Build history of the part. All positions in model axes, mm. A direction names the side the tool comes from. Give positions to 0.01 mm unless a question says otherwise; leave off trailing zeros. Loops run counter-clockwise (first coordinate to the right, second up) from the corner with the lowest first, then second, coordinate; pieces in that order, holes last. Notation, with made-up numbers: (21, 40) -> (79, 40) arc R23 ccw to (79, 69) -> close; hole circle Ø3 at (-38, -36). An arc over 180 degrees is marked (long way). Answer as a JSON object with one key per item and string values. Group by question number.
from build123d import *

# Parameters (mm, degrees)
F0_W     = 7.62
F0_H     = 35.56
F1_DEPTH = 10.795
F0_W_2   = 13.335
F2_DEPTH = 6.35
F3_DEPTH = 10.795
F4_DEPTH = 30.48
F5_R     = 3.81
F6_SIZE  = 16.51
F7_R     = 1.524
F8_DEPTH = 76.836
F9_R     = 3.81


# Not quite as in the source:
# - a feature names something its author has since deleted; it is built from what else it names


with BuildPart() as f1:
    # F0 (on Top) → F1 (new body, symmetric)
    with BuildSketch(Plane.XY):
        Polygon((31.75, 44.45), (-31.75, 44.45), (-31.75, 17.78), (-31.75, -17.78), (-31.75, -44.45), (-29.21, -44.45), (31.75, -44.45), (31.75, -31.7187323975), (31.75, -17.78), (31.75, 17.78), align=None)
        with Locations((-25.4, 0)):
            Rectangle(F0_W, F0_H, mode=Mode.SUBTRACT)
        with Locations((25.4, 0)):
            Rectangle(F0_W, F0_H, mode=Mode.SUBTRACT)
    extrude(amount=F1_DEPTH, both=True)



with BuildPart() as f1b:
    # F0 (on Top) → F1, piece 2 (new body, symmetric)
    with BuildSketch(Plane.XY):
        Polygon((-45.085, -17.78), (-45.085, 17.78), (-45.085, 44.45), (-47.625, 44.45), (-47.625, -31.75), (-47.625, -44.45), (-45.085, -44.45), align=None)
    extrude(amount=F1_DEPTH, both=True)


with BuildPart() as f1c:
    # F0 (on Top) → F1, piece 3 (new body, symmetric)
    with BuildSketch(Plane.XY):
        Polygon((45.085, 44.45), (45.085, 17.78), (45.085, -17.78), (45.085, -44.45), (47.625, -44.45), (47.625, -31.75), (47.625, 44.45), align=None)
    extrude(amount=F1_DEPTH, both=True)


with BuildPart() as f1_1:
    add(f1.part)

    add(f1b.part)  # F2 merges F1b

    add(f1c.part)  # F2 merges F1c
    # F0 (on Top) → F2 (join, symmetric)
    with BuildSketch(Plane.XY):
        with Locations((-38.4175, 0)):
            Rectangle(F0_W_2, F0_H)
        with Locations((38.4175, 0)):
            Rectangle(F0_W_2, F0_H)
    extrude(amount=F2_DEPTH, both=True)

    # F0 (on Top) → F3 (join)
    with BuildSketch(Plane.XY):
        with Locations((25.4, 0)):
            Rectangle(F0_W, F0_H)
        with Locations((-25.4, 0)):
            Rectangle(F0_W, F0_H)
    extrude(amount=-F3_DEPTH)

    # F0 (on Top) → F4 (join)
    with BuildSketch(Plane.XY):
        with Locations((25.4, 0)):
            Rectangle(F0_W, F0_H)
        with Locations((-25.4, 0)):
            Rectangle(F0_W, F0_H)
    extrude(amount=F4_DEPTH)

    # F5
    f5_edges = [f1_1.edges().sort_by_distance(p)[0] for p in [
        (38.4175, -17.78, 6.35),
        (38.4175, -17.78, -6.35),
        (38.4175, 17.78, 6.35),
        (38.4175, 17.78, -6.35),
        (-38.4175, 17.78, -6.35),
        (-38.4175, -17.78, -6.35),
        (-38.4175, 17.78, 6.35),
        (-38.4175, -17.78, 6.35),
    ]]
    fillet(f5_edges, radius=F5_R)

    # F6
    f6_edges = [f1_1.edges().sort_by_distance(p)[0] for p in [
        (25.4, 17.78, 30.48),
        (-25.4, 17.78, 30.48),
        (25.4, -17.78, 30.48),
        (-25.4, -17.78, 30.48),
    ]]
    chamfer(f6_edges, length=F6_SIZE)

    # F7 (on face) → F8 (cut, through all)
    with BuildSketch(Plane.YZ.offset(29.21)):
        with Locations((0, 24.4627408683)):
            Circle(F7_R)
    extrude(amount=-F8_DEPTH, mode=Mode.SUBTRACT)

    # F9
    f9_edges = [f1_1.edges().sort_by_distance(p)[0] for p in [
        (46.355, 44.45, 10.795),
        (-46.355, 44.45, 10.795),
        (-46.355, 44.45, -10.795),
        (46.355, 44.45, -10.795),
        (-46.355, -44.45, 10.795),
        (-46.355, -44.45, -10.795),
        (46.355, -44.45, -10.795),
        (46.355, -44.45, 10.795),
    ]]
    fillet(f9_edges, radius=F9_R)


solid = f1_1.part
(1) Pull direction X, two halves, no side cores. Call faces 4 (the flat face through (-47.625, 1, 0)), 5 (the cylindrical face through (-46.34, -43.3, -9.71)), 6 (the flat face through (38, 0, 6.35)): pulls with the +X half, pulls with the -X half, needs draft (parallel to the pull), parting line crosses it, or undercut.
(2) 3-axis set-ups, long thin cutter, end or side, ignore diameter. For faces 1 (the flat face through (25, 17.78, 12)), 2 (the flat face through (-39, -17.78, 0)), 3 (the cylindrical face through (46.337, 43.364, 9.649)): which of +Z, -Z, +X, -X, +Y, -Y reach the whole face in a straight line?
(3) Probe line 1 along X through (y, z) = (-0.5, -9) (3 decimals); line 2 along Z through (x, y) = (-25.25, 0) (3 decimals). List the from-to ranges inside material, lowest first. Write a range as [from, to].
(4) Saw through at B-B on y = -38. List the corners of the cut face in (x, z) (3 decimals).
(5) Saw through at D-D on x = -13.5. List the corners of the cut face in (y, z) (3 decimals).
(6) Saw through at C-C on y = 7. List the corners of the cut face in (x, z) (3 decimals), plus the area to 3 significant figures.
(7) Pin check, flat tips, straight feed: pin 1 (4 mm diameter, centred on x = -36.5, y = 3.5, fed in from +Z); pin 2 (5.5 mm diameter, centred on x = -41, z = 0, fed in from -Y); pin 3 (10 mm diameter, centred on y = -7.5, z = 18.5, fed in from -X); pin 4 (1.8 mm diameter, centred on y = 0, z = 24.46, fed in from -X). Stop position of each tip, or through.
(8) Saw through at A-A on z = 18. List the corners of the cut face in (x, y).
Calculated:
{
 "1": {"face 4": "pulls with the -X half", "face 5": "needs draft", "face 6": "undercut"},
 "2": {"face 1": "+Z, +X, -X, +Y", "face 2": "+Z, -Z, -Y", "face 3": "+Z, +X, +Y"},
 "3": {"line 1": "x = [-47.625, -45.085], [-31.75, 31.75], [45.085, 47.625]", "line 2": "z = [-10.795, 22.939], [25.987, 30.48]"},
 "4": {"outline": "(-47.625, -10.795) -> (-45.085, -10.795) -> (-45.085, 10.795) -> (-47.625, 10.795) -> close; (-31.75, -10.795) -> (31.75, -10.795) -> (31.75, 10.795) -> (-31.75, 10.795) -> close; (45.085, -10.795) -> (47.625, -10.795) -> (47.625, 10.795) -> (45.085, 10.795) -> close"},
 "5": {"outline": "(-44.45, -10.795) -> (44.45, -10.795) -> (44.45, 10.795) -> (-44.45, 10.795) -> close"},
 "6": {"outline": "(-47.625, -10.795) -> (-45.085, -10.795) -> (-45.085, -6.35) -> (-31.75, -6.35) -> (-31.75, -10.795) -> (31.75, -10.795) -> (31.75, -6.35) -> (45.085, -6.35) -> (45.085, -10.795) -> (47.625, -10.795) -> (47.625, 10.795) -> (45.085, 10.795) -> (45.085, 6.35) -> (31.75, 6.35) -> (31.75, 10.795) -> (29.21, 10.795) -> (29.21, 24.75) -> (21.59, 24.75) -> (21.59, 10.795) -> (-21.59, 10.795) -> (-21.59, 24.75) -> (-29.21, 24.75) -> (-29.21, 10.795) -> (-31.75, 10.795) -> (-31.75, 6.35) -> (-45.085, 6.35) -> (-45.085, 10.795) -> (-47.625, 10.795) -> close", "area": "2,030 mm^2"},
 "7": {"pin 1": "stops at z = 6.35", "pin 2": "stops at y = -17.78", "pin 3": "stops at x = -29.21", "pin 4": "passes through"},
 "8": {"outline": "(-29.21, -13.75) -> (-21.59, -13.75) -> (-21.59, 13.75) -> (-29.21, 13.75) -> close; (21.59, -13.75) -> (29.21, -13.75) -> (29.21, 13.75) -> (21.59, 13.75) -> close"}
}
